Geometry check sheet. Reference: the model listing, model coordinates, mm. A direction names the side the tool comes from. Round coordinates to 2 decimals unless told otherwise and drop trailing zeros. Write each loop counter-clockwise with the first axis right and the second up, starting at its lowest first coordinate (ties: lowest second). Pieces come first, ordered by that corner, then holes.
from build123d import *

# Parameters (mm, degrees)
SKETCH_1_R          = 1.55
SKETCH_1_R_2        = 1.05
EXTRUDE_1_DEPTH     = 6
SKETCH_2_R          = 1.05
CUT_EXTRUDE_1_DEPTH = 31.777426793
SKETCH_3_R          = 4
CUT_EXTRUDE_2_DEPTH = 3


with BuildPart() as part:
    # ｽｹｯﾁ1 → ﾎﾞｽ - 押し出し1 (new body)
    with BuildSketch(Plane(origin=(0, 0, 0), x_dir=(1, 0, 0), z_dir=(0, 1, 0))):
        with BuildLine():
            Line((-10, 13.5), (10, 13.5))
            ThreePointArc((10, 13.5), (12.474873734, 12.474873734), (13.5, 10))
            Line((13.5, 10), (13.5, -10))
            ThreePointArc((13.5, -10), (12.474873734, -12.474873734), (10, -13.5))
            Line((10, -13.5), (-10, -13.5))
            ThreePointArc((-10, -13.5), (-12.474873734, -12.474873734), (-13.5, -10))
            Line((-13.5, -10), (-13.5, 10))
            ThreePointArc((-13.5, 10), (-12.474873734, 12.474873734), (-10, 13.5))
        make_face()
        with Locations(Location((0, 0, 0), (0, 0, 270))):
            Circle(SKETCH_1_R, mode=Mode.SUBTRACT)
        with Locations(Location((-10.5, -10.5, 0), (0, 0, 270))):
            Circle(SKETCH_1_R_2, mode=Mode.SUBTRACT)
        with Locations(Location((10.5, -10.5, 0), (0, 0, 270))):
            Circle(SKETCH_1_R_2, mode=Mode.SUBTRACT)
        with Locations(Location((10.5, 10.5, 0), (0, 0, 270))):
            Circle(SKETCH_1_R_2, mode=Mode.SUBTRACT)
        with Locations(Location((-10.5, 10.5, 0), (0, 0, 270))):
            Circle(SKETCH_1_R_2, mode=Mode.SUBTRACT)
    extrude(amount=EXTRUDE_1_DEPTH)

    # ｽｹｯﾁ2 → ｶｯﾄ - 押し出し1 (cut, through all)
    with BuildSketch(Plane(origin=(13.5, 0, 0), x_dir=(0, 0, -1), z_dir=(1, 0, 0))):
        with Locations((0, 3)):
            Circle(SKETCH_2_R)
    extrude(amount=-CUT_EXTRUDE_1_DEPTH, mode=Mode.SUBTRACT)

    # ｽｹｯﾁ3 → ｶｯﾄ - 押し出し2 (cut)
    with BuildSketch(Plane.XZ):
        with Locations(Location((0, 0, 0), (0, 0, 270))):
            Circle(SKETCH_3_R)
    extrude(amount=-CUT_EXTRUDE_2_DEPTH, mode=Mode.SUBTRACT)


solid = part.part
1. Release check for a two-part mould opening along X. For faces 3 (the face through (10.82, 2.96, 11.5)), 4 (the face through (3, 6, 0)), 5 (the face through (12.5, 2.96, 12.45)) record: +X half, -X half, draft (parallel to the pull), parting line (faces both ways), or undercut.
2. Section check A-A (y = 2.5). Record the cut outline in (x, z), plus the area to 3 significant figures.
3. Section check C-C (z = 0). Record the cut outline in (x, y).
4. Access from +Z, -Z, +X, -X, +Y, -Y to the whole of each face (thin tool, end or side, straight path). Record for faces 1 (the face through (-3.549, 1.479, -1.846)), 2 (the face through (-9.61, 2.96, -9.94)).
5. Depth check by flat-ended pin: pin 1 Ø1.9 at (y, z) = (3, 0) entering from -X. Enter the tip coordinate at first touch or a pass-through.
6. Section check B-B (x = 0). Record the cut outline in (y, z).
7. Scan lines: line 1 along X through (y, z) = (4.2, -10.5); line 2 along X through (y, z) = (3, -11); line 3 along Y through (x, z) = (8.75, 0). Record each from-to range of solid material in increasing order.
8. Section check D-D (x = -10.5). Record the cut outline in (y, z), plus the area to 3 significant figures.
Results below:
1. face 3: undercut
1. face 4: draft
1. face 5: +X half
2. outline: (-13.5, -10) arc R3.5 ccw to (-10, -13.5) - (10, -13.5) arc R3.5 ccw to (13.5, -10) - (13.5, -0.92) - (3.89, -0.92) arc R4 cw to (-3.89, -0.92) - (-13.5, -0.92) - close; (-13.5, 0.92) - (-3.89, 0.92) arc R4 cw to (3.89, 0.92) - (13.5, 0.92) - (13.5, 10) arc R3.5 ccw to (10, 13.5) - (-10, 13.5) arc R3.5 ccw to (-13.5, 10) - close; hole circle Ø2.1 at (-10.5, -10.5); hole circle Ø2.1 at (-10.5, 10.5); hole circle Ø2.1 at (10.5, -10.5); hole circle Ø2.1 at (10.5, 10.5)
2. area: 619 mm2
3. outline: (-13.5, 0) - (-4, 0) - (-4, 1.95) - (-13.5, 1.95) - close; (-13.5, 4.05) - (-1.55, 4.05) - (-1.55, 6) - (-13.5, 6) - close; (1.55, 4.05) - (13.5, 4.05) - (13.5, 6) - (1.55, 6) - close; (4, 0) - (13.5, 0) - (13.5, 1.95) - (4, 1.95) - close
4. face 1: -Y
4. face 2: +Y, -Y
5. pin 1: passes through
6. outline: (0, -13.5) - (6, -13.5) - (6, -1.55) - (3, -1.55) - (3, -4) - (0, -4) - close; (0, 4) - (3, 4) - (3, 1.55) - (6, 1.55) - (6, 13.5) - (0, 13.5) - close
7. line 1: x = -13.46 to -11.55, -9.45 to 9.45, 11.55 to 13.46
7. line 2: x = -13.35 to -11.42, -9.58 to 9.58, 11.42 to 13.35
7. line 3: y = 0 to 1.95, 4.05 to 6
8. outline: (0, -13.46) - (6, -13.46) - (6, -11.55) - (0, -11.55) - close; (0, -9.45) - (6, -9.45) - (6, 9.45) - (0, 9.45) - close; (0, 11.55) - (6, 11.55) - (6, 13.46) - (0, 13.46) - close; hole circle Ø2.1 at (3, 0)
8. area: 133 mm2
